Geometry check sheet. Reference: the model listing, model coordinates, mm. Coordinates: 2 decimals unless noted, no trailing zeros. Write each loop counter-clockwise with the first axis right and the second up, starting at its lowest first coordinate (ties: lowest second). Pieces come first, ordered by that corner, then holes. Notation, with made-up numbers: (-24, -33) -> (-20, -33) arc R11 ccw to (-20, -13) -> close; hole circle Ø7 at (-8.5, -6). An arc over 180 degrees is marked (long way). Answer in a Markdown table with one row per item. Add a question column.
Q1. Section check A-A, the plane y = 0. Record the boundary of the cut face in (x, z).
Q2. Gauge pin test, flat end, axial feed: P1, Ø1, axis at x = 18, z = 1.5, coming from the +Y side. Record the tip position at first contact, or that the pin passes through.
Q3. Section check B-B, the plane z = 0.85. Record the boundary of the cut face in (x, y), and give its area (3 significant figures).
Q4. Thickness scan on line 1 (Y direction, x = 0, z = 1.4); line 2 (Y direction, x = 60, z = 1.25); line 3 (Y direction, x = -24.5, z = 2.2). Record the ranges inside material, lowest first.
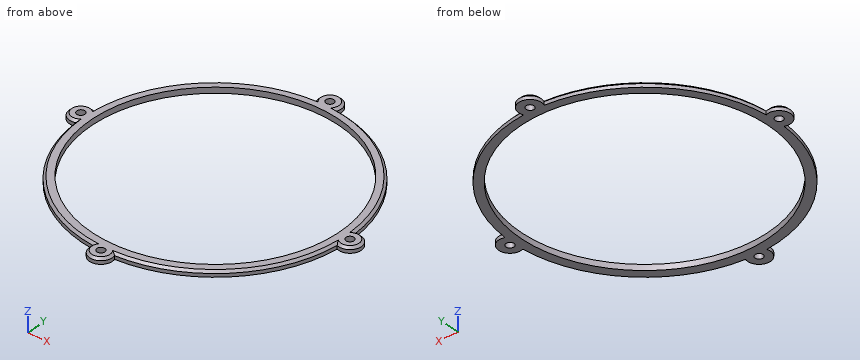
```python
from build123d import *

# Parameters (mm, degrees)
SKETCH_R     = 54.5
SKETCH_R_2   = 1.75
PAD_DEPTH    = 2.5
CHAMFER_SIZE = 1


with BuildPart() as part:
    # Sketch → Pad (new body)
    with BuildSketch(Plane.XY):
        with BuildLine():
            ThreePointArc((4.584354, 58.00408), (-0.000818, 65), (-4.583701, 58.00258))
            ThreePointArc((-4.583701, 58.00258), (-41.189101, 41.181927), (-58.202656, 4.665785))
            ThreePointArc((-58.202656, 4.665785), (-64.999962, 0.019578), (-58.239249, -4.679717))
            ThreePointArc((-58.239249, -4.679717), (-41.41212, -41.428831), (-4.756492, -58.458643))
            ThreePointArc((-4.756492, -58.458643), (-0.000824, -65), (4.757, -58.460212))
            ThreePointArc((4.757, -58.460212), (41.4225, -41.438205), (58.258407, -4.686881))
            ThreePointArc((58.258407, -4.686881), (64.999962, 0.019584), (58.221745, 4.673094))
            ThreePointArc((58.221745, 4.673094), (41.19943, 41.191251), (4.584354, 58.00408))
        make_face()
        Circle(SKETCH_R, mode=Mode.SUBTRACT)
        with Locations((0, 60)):
            Circle(SKETCH_R_2, mode=Mode.SUBTRACT)
        with Locations((0, -60)):
            Circle(SKETCH_R_2, mode=Mode.SUBTRACT)
        with Locations((-60, 0)):
            Circle(SKETCH_R_2, mode=Mode.SUBTRACT)
        with Locations((60, 0)):
            Circle(SKETCH_R_2, mode=Mode.SUBTRACT)
    extrude(amount=PAD_DEPTH)

    # Chamfer
    chamfer_edges = [part.edges().sort_by_distance(p)[0] for p in [
        (41.4225, -41.438205, 2.5),
        (-0.000824, -65, 2.5),
        (-41.41212, -41.428831, 2.5),
        (-64.999962, 0.019578, 2.5),
        (-41.189101, 41.181927, 2.5),
        (64.999962, 0.019584, 2.5),
        (41.19943, 41.191251, 2.5),
        (-0.000818, 65, 2.5),
    ]]
    chamfer(chamfer_edges, length=CHAMFER_SIZE)


solid = part.part
```
Calculated:
| question | item | result |
|---|---|---|
| 1 | outline | (-65, 0) -> (-61.75, 0) -> (-61.75, 2.5) -> (-64, 2.5) -> (-65, 1.5) -> close; (-58.25, 0) -> (-54.5, 0) -> (-54.5, 2.5) -> (-58.25, 2.5) -> close; (54.5, 0) -> (58.25, 0) -> (58.25, 2.5) -> (54.5, 2.5) -> close; (61.75, 0) -> (65, 0) -> (65, 1.5) -> (64, 2.5) -> (61.75, 2.5) -> close |
| 2 | P1 | stops at y = 55.5 |
| 3 | outline | (-58.24, -4.68) arc R58.42 ccw to (-4.76, -58.46) arc R5 ccw (long way) to (4.76, -58.46) arc R58.42 ccw to (58.26, -4.69) arc R5 ccw (long way) to (58.22, 4.67) arc R58.42 ccw to (4.58, 58) arc R5 ccw (long way) to (-4.58, 58) arc R58.42 ccw to (-58.2, 4.67) arc R5 ccw (long way) to start; hole circle Ø3.5 at (-60, 0); hole circle Ø109 at (0, 0); hole circle Ø3.5 at (0, -60); hole circle Ø3.5 at (0, 60); hole circle Ø3.5 at (60, 0) |
| 3 | area | 1,570 mm² |
| 4 | line 1 | y = -65 to -61.75, -58.25 to -54.5, 54.5 to 58.25, 61.75 to 65 |
| 4 | line 2 | y = -5 to -1.75, 1.75 to 5 |
| 4 | line 3 | y = -52.49 to -48.68, 48.68 to 52.02 |
